Verification items for the finished model (mm, model axes). A direction names the side the tool comes from. Coordinates: 2 decimals unless noted, no trailing zeros. Order: outer loops, then holes, each group sorted by start corner. A loop starts at its lowest first (then second) coordinate and runs counter-clockwise, first axis right, second up. Notation, with made-up numbers: M 48.5,11.25 L 60.5,11.25 A3 cw 60.5,16.25 Z; hole C 37,16.5 d4. An arc over 180 degrees is marked long. Answer as a JSON object with one key per item and string values. Group by question number.
(1) Material ranges on line 1 (X direction, y = 1.15, z = 159); line 2 (Z direction, x = 0.8, y = 8), recorded low to high.
(2) Gauge pin test, flat ends, axial feed: pin 1 Ø3.5 at (x, z) = (7, 454) entering from +Y; pin 2 Ø1 at (x, y) = (2, 8.5) entering from +Z; pin 3 Ø6.5 at (x, z) = (6.5, 276.5) entering from +Y; pin 4 Ø7 at (y, z) = (7, 10) entering from +X. Record the tip position at first contact, or that the pin passes through.
(3) Access from +Z, -Z, +X, -X, +Y, -Y to the whole of each face (thin tool, end or side, straight path). Record for faces 1 (the face through (1, 9, 459)), 2 (the face through (8, 2, 229)).
(4) Cross-section at A-A (z = 111). Enter the section's corners in (x, y).
from build123d import *

# Parameters (mm, degrees)
EXTRUDE_1_DEPTH            = 464
CHAMFER_1_SIZE             = 11
HOLE_WIZARD_M41_AT_2_COUNT = 2
HOLE_WIZARD_M41_AT_2_PITCH = 407
HOLE_WIZARD_M51_AT_2_COUNT = 2
HOLE_WIZARD_M51_AT_2_PITCH = 138
HOLE_WIZARD_M51_AT_3_COUNT = 2
HOLE_WIZARD_M51_AT_3_PITCH = 276
HOLE_WIZARD_M51_AT_4_COUNT = 2
HOLE_WIZARD_M51_AT_4_PITCH = 414
HOLE_WIZARD_M52_AT_2_COUNT = 2
HOLE_WIZARD_M52_AT_2_PITCH = 138
HOLE_WIZARD_M52_AT_3_COUNT = 2
HOLE_WIZARD_M52_AT_3_PITCH = 276
HOLE_WIZARD_M52_AT_4_COUNT = 2
HOLE_WIZARD_M52_AT_4_PITCH = 414


with BuildPart() as part:
    # Эскиз1 → Бобышка-Вытянуть1 (new body)
    with BuildSketch(Plane.XY):
        Polygon((0, 0), (0, 15), (2, 15), (2, 2), (15, 2), (15, 0), align=None)
    extrude(amount=EXTRUDE_1_DEPTH)

    # Фаска1
    chamfer_1_edges = [part.edges().sort_by_distance(p)[0] for p in [
        (1, 15, 464),
        (1, 15, 0),
        (15, 1, 464),
        (15, 1, 0),
    ]]
    chamfer(chamfer_1_edges, length=CHAMFER_1_SIZE)

    # Эскиз2 → Зенковка для винта с потайной головкой M41 (revolve, cut)
    with BuildSketch(Plane(origin=(7, 0, 454), x_dir=(0, 0, -1), z_dir=(1, 0, 0))):
        Polygon((0, 0), (0, 2), (2.4, 2), (2.25, 1.85), (2.25, 1.45), (3.7, 0), align=None)
    hole_wizard_m41 = revolve(axis=Axis((7, -6.35, 454), (0, 1, 0)), mode=Mode.SUBTRACT)

    # Зенковка для винта с потайной головкой M41 at 2: Зенковка для винта с потайной головкой M41 ×2
    with Locations(*[(0, 0, -i * HOLE_WIZARD_M41_AT_2_PITCH) for i in range(1, HOLE_WIZARD_M41_AT_2_COUNT)]):
        add(hole_wizard_m41, mode=Mode.SUBTRACT)

    # Эскиз6 → Зенковка для винта с потайной головкой M42 (revolve, cut)
    with BuildSketch(Plane(origin=(0, 7, 10), x_dir=(0, 0, 1), z_dir=(0, 1, 0))):
        Polygon((0, 0), (0, 2), (2.4, 2), (2.25, 1.85), (2.25, 1.45), (3.7, 0), align=None)
    revolve(axis=Axis((-6.35, 7, 10), (1, 0, 0)), mode=Mode.SUBTRACT)

    # Эскиз8 → Отверстие с зазором M51 (revolve, cut)
    with BuildSketch(Plane(origin=(0, 8, 29), x_dir=(0, 0, 1), z_dir=(0, 1, 0))):
        Polygon((0, 0), (0, 2), (3, 2), (2.9, 1.9), (2.9, 0.1), (3, 0), align=None)
    hole_wizard_m51 = revolve(axis=Axis((-6.35, 8, 29), (1, 0, 0)), mode=Mode.SUBTRACT)

    # Отверстие с зазором M51 at 2: Отверстие с зазором M51 ×2
    with Locations(*[(0, 0, i * HOLE_WIZARD_M51_AT_2_PITCH) for i in range(1, HOLE_WIZARD_M51_AT_2_COUNT)]):
        add(hole_wizard_m51, mode=Mode.SUBTRACT)

    # Отверстие с зазором M51 at 3: Отверстие с зазором M51 ×2
    with Locations(*[(0, 0, i * HOLE_WIZARD_M51_AT_3_PITCH) for i in range(1, HOLE_WIZARD_M51_AT_3_COUNT)]):
        add(hole_wizard_m51, mode=Mode.SUBTRACT)

    # Отверстие с зазором M51 at 4: Отверстие с зазором M51 ×2
    with Locations(*[(0, 0, i * HOLE_WIZARD_M51_AT_4_PITCH) for i in range(1, HOLE_WIZARD_M51_AT_4_COUNT)]):
        add(hole_wizard_m51, mode=Mode.SUBTRACT)

    # Эскиз10 → Отверстие с зазором M52 (revolve, cut)
    with BuildSketch(Plane(origin=(8, 0, 21), x_dir=(0, 0, -1), z_dir=(1, 0, 0))):
        Polygon((0, 0), (0, 2), (3, 2), (2.9, 1.9), (2.9, 0.1), (3, 0), align=None)
    hole_wizard_m52 = revolve(axis=Axis((8, -6.35, 21), (0, 1, 0)), mode=Mode.SUBTRACT)

    # Отверстие с зазором M52 at 2: Отверстие с зазором M52 ×2
    with Locations(*[(0, 0, i * HOLE_WIZARD_M52_AT_2_PITCH) for i in range(1, HOLE_WIZARD_M52_AT_2_COUNT)]):
        add(hole_wizard_m52, mode=Mode.SUBTRACT)

    # Отверстие с зазором M52 at 3: Отверстие с зазором M52 ×2
    with Locations(*[(0, 0, i * HOLE_WIZARD_M52_AT_3_PITCH) for i in range(1, HOLE_WIZARD_M52_AT_3_COUNT)]):
        add(hole_wizard_m52, mode=Mode.SUBTRACT)

    # Отверстие с зазором M52 at 4: Отверстие с зазором M52 ×2
    with Locations(*[(0, 0, i * HOLE_WIZARD_M52_AT_4_PITCH) for i in range(1, HOLE_WIZARD_M52_AT_4_COUNT)]):
        add(hole_wizard_m52, mode=Mode.SUBTRACT)


solid = part.part
Taken from the geometry:
{
 "1": {"line 1": "x = 0 to 5.1, 10.9 to 15", "line 2": "z = 4 to 7.28, 12.72 to 26.1, 31.9 to 164.1, 169.9 to 302.1, 307.9 to 440.1, 445.9 to 460"},
 "2": {"pin 1": "passes through", "pin 2": "stops at z = 460", "pin 3": "stops at y = 2", "pin 4": "stops at x = 2"},
 "3": {"face 1": "+Z, +X, -X, +Y", "face 2": "+Z, -Z, +X, +Y"},
 "4": {"outline": "M 0,0 L 15,0 L 15,2 L 2,2 L 2,15 L 0,15 Z"}
}
